from build123d import *

# Parameters (mm, degrees)
SKETCH1_W           = 191
SKETCH1_H           = 163
BOSS_EXTRUDE1_DEPTH = 20
FILLET1_R           = 10
FILLET2_R           = 5
SHELL1_T            = -2
SKETCH2_R           = 3
CUT_EXTRUDE1_DEPTH  = 10


with BuildPart() as part:
    # Sketch1 → Boss-Extrude1 (new body)
    with BuildSketch(Plane.XY):
        Rectangle(SKETCH1_W, SKETCH1_H)
    extrude(amount=BOSS_EXTRUDE1_DEPTH)

    # Fillet1
    fillet1_edges = [part.edges().sort_by_distance(p)[0] for p in [
        (95.5, -81.5, 10),
        (-95.5, -81.5, 10),
        (-95.5, 81.5, 10),
        (95.5, 81.5, 10),
    ]]
    fillet(fillet1_edges, radius=FILLET1_R)

    # Fillet2
    fillet2_edges = [part.edges().sort_by_distance(p)[0] for p in [
        (0, -81.5, 20),
        (-95.5, 0, 20),
        (95.5, 0, 20),
        (0, 81.5, 20),
        (-92.571067812, 78.571067812, 20),
        (92.571067812, 78.571067812, 20),
        (92.571067812, -78.571067812, 20),
        (-92.571067812, -78.571067812, 20),
    ]]
    fillet(fillet2_edges, radius=FILLET2_R)

    # Shell1
    shell1_openings = [part.faces().sort_by_distance(p)[0] for p in [
        (0, 0, 0),
    ]]
    offset(amount=SHELL1_T, openings=shell1_openings, kind=Kind.INTERSECTION)

    # Sketch2 → Cut-Extrude1 (cut)
    with BuildSketch(Plane(origin=(0, 0, 18), x_dir=(-1, 0, 0), z_dir=(0, 0, -1))):
        Circle(SKETCH2_R)
    extrude(amount=-CUT_EXTRUDE1_DEPTH, mode=Mode.SUBTRACT)


solid = part.part
Verification items for the finished model (mm, model axes). A direction names the side the tool comes from. Coordinates: 2 decimals unless noted, no trailing zeros. Write each loop counter-clockwise with the first axis right and the second up, starting at its lowest first coordinate (ties: lowest second). Pieces come first, ordered by that corner, then holes. Notation, with made-up numbers: M 2,70 L 36,70 A6 ccw 36,79 Z; hole C 85,-29 d3. An arc over 180 degrees is marked long. Use a Markdown table: item, result.
Q1. Set-up check for faces 4 (the face through (-91.219, -77.094, 7.605)), 5 (the face through (95.5, -1, 7)): record each of +Z, -Z, +X, -X, +Y, -Y from which the full face is reachable in a straight line by a thin tool's end or side.
Reply:
| item | result |
|---|---|
| face 4 | -Z |
| face 5 | +Z, -Z, +X, +Y, -Y |
Q2. Thickness scan on line 1 (Y direction, x = -43.5, z = 8.75); line 2 (X direction, y = -64, z = 5.25); line 3 (Z direction, x = -80, y = -72.5). Record the ranges inside material, lowest first.
Reply:
| item | result |
|---|---|
| line 1 | y = -81.5 to -79.5, 79.5 to 81.5 |
| line 2 | x = -95.5 to -93.5, 93.5 to 95.5 |
| line 3 | z = 18 to 20 |
Q3. Sectioned sample at D-D, the plane y = -67. Record the boundary of the cut face in (x, z), plus the area to 3 significant figures.
Reply:
| item | result |
|---|---|
| outline | M -95.5,0 L -93.5,0 L -93.5,15 A3 cw -90.5,18 L 90.5,18 A3 cw 93.5,15 L 93.5,0 L 95.5,0 L 95.5,15 A5 ccw 90.5,20 L -90.5,20 A5 ccw -95.5,15 Z |
| area | 447 mm² |
Q4. Sectioned sample at C-C, the plane z = 12.25. Record the boundary of the cut face in (x, y), plus the area to 3 significant figures.
Reply:
| item | result |
|---|---|
| outline | M -95.5,-71.5 A10 ccw -85.5,-81.5 L 85.5,-81.5 A10 ccw 95.5,-71.5 L 95.5,71.5 A10 ccw 85.5,81.5 L -85.5,81.5 A10 ccw -95.5,71.5 Z; hole M -93.5,-71.5 A8 ccw -85.5,-79.5 L 85.5,-79.5 A8 ccw 93.5,-71.5 L 93.5,71.5 A8 ccw 85.5,79.5 L -85.5,79.5 A8 ccw -93.5,71.5 Z |
| area | 1,370 mm² |
Q5. Sectioned sample at A-A, the plane y = 0. Record the boundary of the cut face in (x, z).
Reply:
| item | result |
|---|---|
| outline | M -95.5,0 L -93.5,0 L -93.5,15 A3 cw -90.5,18 L -3,18 L -3,20 L -90.5,20 A5 ccw -95.5,15 Z; M 3,18 L 90.5,18 A3 cw 93.5,15 L 93.5,0 L 95.5,0 L 95.5,15 A5 ccw 90.5,20 L 3,20 Z |
Q6. Draft check along Y on faces 1 (the face through (-95.5, -1, 7)), 2 (the face through (-1, 79.5, 7)), 3 (the face through (-1, -81.5, 7)). Enter one of: +Y half, -Y half, draft (parallel to the pull), parting line (faces both ways), or undercut.
Reply:
| item | result |
|---|---|
| face 1 | draft |
| face 2 | undercut |
| face 3 | -Y half |
Q7. Go/stop test with a flat-tipped pin: P1, Ø3, axis at x = -52.5, y = 8, coming from the -Z side. Record where the tip stops, or that it passes through.
Reply:
| item | result |
|---|---|
| P1 | stops at z = 18 |
Q8. Sectioned sample at B-B, the plane x = 0. Record the boundary of the cut face in (y, z).
Reply:
| item | result |
|---|---|
| outline | M -81.5,0 L -79.5,0 L -79.5,15 A3 cw -76.5,18 L -3,18 L -3,20 L -76.5,20 A5 ccw -81.5,15 Z; M 3,18 L 76.5,18 A3 cw 79.5,15 L 79.5,0 L 81.5,0 L 81.5,15 A5 ccw 76.5,20 L 3,20 Z |
